```python
from build123d import *

# Parameters (mm, degrees)
SKETCH1_W          = 98.9
SKETCH1_H          = 124.45
BODY_DEPTH         = 22.55
SKETCH4_W          = 7
SKETCH4_H          = 3
SKETCH4_W_2        = 3
SKETCH4_H_2        = 7
CUT_EXTRUDE1_DEPTH = 63
SKETCH5_W          = 8.299397568
SKETCH5_H          = 10.9
CUT_EXTRUDE2_DEPTH = 63
SKETCH6_W          = 98.9
SKETCH6_H          = 68.5
CUT_EXTRUDE3_DEPTH = 63
SKETCH7_W          = 22.55
SKETCH7_H          = 1.441759006
CUT_EXTRUDE4_DEPTH = 63
CUT_EXTRUDE5_DEPTH = 23.55
SKETCH9_R          = 1.25
CUT_EXTRUDE6_DEPTH = 10


with BuildPart() as part:
    # Sketch1 → body (new body)
    with BuildSketch(Plane.XY):
        Rectangle(SKETCH1_W, SKETCH1_H)
    extrude(amount=BODY_DEPTH)

    # Sketch4 → Cut-Extrude1 (cut)
    with BuildSketch(Plane(origin=(0, 0, 0), x_dir=(-1, 0, 0), z_dir=(0, 0, -1))):
        with Locations((0, 62.225)):
            Rectangle(SKETCH4_W, SKETCH4_H)
        with Locations((49.35, 12.775)):
            Rectangle(SKETCH4_W_2, SKETCH4_H_2)
        with Locations((-49.45, 12.875)):
            Rectangle(SKETCH4_W_2, SKETCH4_H_2)
    extrude(amount=-CUT_EXTRUDE1_DEPTH, mode=Mode.SUBTRACT)

    # Sketch5 → Cut-Extrude2 (cut)
    with BuildSketch(Plane(origin=(0, 0, 0), x_dir=(-1, 0, 0), z_dir=(0, 0, -1))):
        with Locations((-0.05, 12.825)):
            Rectangle(SKETCH5_W, SKETCH5_H)
        with BuildLine():
            Line((4.099698784, 18.275), (4.099698784, 7.375))
            ThreePointArc((4.099698784, 7.375), (6.087912376, 9.783860137), (6.8, 12.825))
            ThreePointArc((6.8, 12.825), (6.087912376, 15.866139863), (4.099698784, 18.275))
        make_face()
        with BuildLine():
            ThreePointArc((-4.199698784, 18.275), (-6.9, 12.825), (-4.199698784, 7.375))
            Line((-4.199698784, 7.375), (-4.199698784, 18.275))
        make_face()
    extrude(amount=-CUT_EXTRUDE2_DEPTH, mode=Mode.SUBTRACT)

    # Sketch6 → Cut-Extrude3 (cut)
    with BuildSketch(Plane(origin=(0, 0, 0), x_dir=(-1, 0, 0), z_dir=(0, 0, -1))):
        with BuildLine():
            Line((49.45, 19.275), (49.45, 62.225))
            Line((49.45, 62.225), (6.5, 62.225))
            Line((6.5, 62.225), (6.5, 22.275))
            ThreePointArc((6.5, 22.275), (8.621320344, 21.396320344), (9.5, 19.275))
            Line((9.5, 19.275), (49.45, 19.275))
        make_face()
        with BuildLine():
            Line((-49.45, 60.783244994), (-49.45, 19.391375139))
            Line((-49.45, 19.391375139), (-9.597617792, 19.297494249))
            ThreePointArc((-9.597617792, 19.297494249), (-8.71394336, 21.416738793), (-6.590558988, 22.290418797))
            Line((-6.590558988, 22.290418797), (-6.496484462, 62.225))
            Line((-6.496484462, 62.225), (-49.446603635, 62.225))
            Line((-49.446603635, 62.225), (-49.45, 60.783244994))
        make_face()
        with Locations((0, -27.975)):
            Rectangle(SKETCH6_W, SKETCH6_H)
    extrude(amount=-CUT_EXTRUDE3_DEPTH, mode=Mode.SUBTRACT)

    # Sketch7 → Cut-Extrude4 (cut)
    with BuildSketch(Plane(origin=(49.592912844, 0.116826812, 0), x_dir=(0, 0, 1), z_dir=(-0.999997225, -0.002355709, 0))):
        with Locations((11.275, 61.387466016)):
            Rectangle(SKETCH7_W, SKETCH7_H)
    extrude(amount=-CUT_EXTRUDE4_DEPTH, mode=Mode.SUBTRACT)

    # Sketch8 → Cut-Extrude5 (cut, through all)
    with BuildSketch(Plane.XY.offset(22.55)):
        with BuildLine():
            Line((-49.45, 6.275), (-17.5, 6.275))
            Line((-17.5, 6.275), (-17.5, 12.825))
            Line((-17.5, 12.825), (-6.8, 12.825))
            ThreePointArc((-6.8, 12.825), (-6.087912376, 15.866139863), (-4.099698784, 18.275))
            Line((-4.099698784, 18.275), (4.199698784, 18.275))
            ThreePointArc((4.199698784, 18.275), (6.187912376, 15.866139863), (6.9, 12.825))
            Line((6.9, 12.825), (17.5, 12.825))
            Line((17.5, 12.825), (17.5, 6.275))
            Line((17.5, 6.275), (49.45, 6.275))
            Line((49.45, 6.275), (49.45, 9.375))
            Line((49.45, 9.375), (47.95, 9.375))
            Line((47.95, 9.375), (47.95, 16.375))
            Line((47.95, 16.375), (49.45, 16.375))
            Line((49.45, 16.375), (49.45, 19.391375139))
            Line((49.45, 19.391375139), (9.597617792, 19.297494249))
            ThreePointArc((9.597617792, 19.297494249), (8.71394336, 21.416738793), (6.590558988, 22.290418797))
            Line((6.590558988, 22.290418797), (6.496484462, 62.225))
            Line((6.496484462, 62.225), (3.5, 62.225))
            Line((3.5, 62.225), (3.5, 60.725))
            Line((3.5, 60.725), (-3.5, 60.725))
            Line((-3.5, 60.725), (-3.5, 62.225))
            Line((-3.5, 62.225), (-6.5, 62.225))
            Line((-6.5, 62.225), (-6.5, 22.275))
            ThreePointArc((-6.5, 22.275), (-8.621320344, 21.396320344), (-9.5, 19.275))
            Line((-9.5, 19.275), (-49.45, 19.275))
            Line((-49.45, 19.275), (-49.45, 16.275))
            Line((-49.45, 16.275), (-47.85, 16.275))
            Line((-47.85, 16.275), (-47.85, 9.275))
            Line((-47.85, 9.275), (-49.45, 9.275))
            Line((-49.45, 9.275), (-49.45, 6.275))
        make_face()
    extrude(amount=-CUT_EXTRUDE5_DEPTH, mode=Mode.SUBTRACT)

    # Sketch9 → Cut-Extrude6 (cut)
    with BuildSketch(Plane.XZ.offset(-6.275)):
        with Locations((13, 11.275)):
            Circle(SKETCH9_R)
        with Locations((-13, 11.275)):
            Circle(SKETCH9_R)
    extrude(amount=-CUT_EXTRUDE6_DEPTH, mode=Mode.SUBTRACT)


solid = part.part
```
Geometry: final body of the model. Coordinates: model frame, mm. A direction names the side the tool comes from. Round coordinates to 2 decimals unless told otherwise and drop trailing zeros. Order: outer loops, then holes, each group sorted by start corner. A loop starts at its lowest first (then second) coordinate and runs counter-clockwise, first axis right, second up. Notation, with made-up numbers: (79.5, -20.5) - (125.5, -20.5) arc R29 ccw to (125.5, 6.5) - close; hole circle Ø9 at (-35, 36). An arc over 180 degrees is marked (long way). Use CSV: the item, a comma, the result in double quotes. Start each with the question number.
Q1. Material intervals for line 1 along Z through (x, y) = (13, 11) (3 decimals); line 2 along X through (y, z) = (11.25, 9.75); line 3 along X through (y, z) = (10.25, 9), sorted ascending. Write a range as from..to.
Q2. Section query C-C (z = 16.25). Return loops of the section in (x, y) (3 decimals).
Q3. Section query D-D (y = 12). Return loops of the section in (x, z) (3 decimals), and give its area (3 significant figures).
Q4. Section query A-A (y = 9.25). Return loops of the section in (x, z) (3 decimals).
Q5. Section query B-B (x = 13). Return loops of the section in (y, z) (3 decimals).
Q6. Mould query, pull axis X, two halves, no side actions, for faces 1 (the face through (-17.5, 10, 11)), 2 (the face through (11, 12.825, 11)), 3 (the face through (17.5, 10, 11)), 4 (the face through (-13.99, 9.5, 10.51)). Classes: +X half, -X half, draft (parallel to the pull), parting line (faces both ways), or undercut.
Q7. Access query for faces 5 (the face through (6.207, 9.823, 11.117)), 6 (the face through (12.729, 9.504, 10.055)). Directions: +Z, -Z, +X, -X, +Y, -Y. A direction counts if a zero-diameter tool reaches every point of the face in a straight line with its end or side. Return the directions, or none.
Q8. First-contact query: pin 1 (2.5 mm diameter, centred on x = 0.5, z = 10, fed in from +Y) (3 decimals); pin 2 (2 mm diameter, centred on x = 13, z = 11.275, fed in from +Y). Flat tips, straight axial feed; report the tip coordinate or a pass-through.
Result set:
1,line 1,"z = 0..10.025, 12.525..22.55"
1,line 2,"x = -17.5..-6.62, 6.72..17.5"
1,line 3,"x = -17.5..-6.3, 6.4..17.5"
2,outline,"(-17.5, 6.275) - (17.5, 6.275) - (17.5, 12.825) - (6.9, 12.825) arc R6.85 cw to (4.2, 7.375) - (-4.1, 7.375) arc R6.85 cw to (-6.8, 12.825) - (-17.5, 12.825) - close"
3,outline,"(-17.5, 0) - (-6.75, 0) - (-6.75, 22.55) - (-17.5, 22.55) - close; (6.85, 0) - (17.5, 0) - (17.5, 22.55) - (6.85, 22.55) - close; hole circle Ø2.5 at (-13, 11.275); hole circle Ø2.5 at (13, 11.275)"
3,area,"473 mm2"
4,outline,"(-17.5, 0) - (-5.793, 0) - (-5.793, 22.55) - (-17.5, 22.55) - close; (5.893, 0) - (17.5, 0) - (17.5, 22.55) - (5.893, 22.55) - close; hole circle Ø2.5 at (-13, 11.275); hole circle Ø2.5 at (13, 11.275)"
5,outline,"(6.275, 0) - (12.825, 0) - (12.825, 10.025) - (6.275, 10.025) - close; (6.275, 12.525) - (12.825, 12.525) - (12.825, 22.55) - (6.275, 22.55) - close"
6,face 1,"-X half"
6,face 2,"draft"
6,face 3,"+X half"
6,face 4,"undercut"
7,face 5,"+Z, -Z, +Y"
7,face 6,"+Y, -Y"
8,pin 1,"stops at y = 7.375"
8,pin 2,"passes through"
